Read the model definition and answer for the solid it produces. Units are mm, in the model's axes. A direction names the side the tool comes from. Give positions to 0.01 mm unless a question says otherwise; leave off trailing zeros. Loops run counter-clockwise (first coordinate to the right, second up) from the corner with the lowest first, then second, coordinate; pieces in that order, holes last.
(1) Each of these flat-tipped pins is pushed along its axis until it touches: P1, Ø2, axis at y = 0, z = 1, coming from the -X side; P2, Ø0.8, axis at x = 0, z = 1.5, coming from the +Y side; P3, Ø3, axis at y = 0, z = 1, coming from the +X side; P4, Ø6.5, axis at x = -1.5, y = 1.5, coming from the -Z side. Where does it stop, or does it pass through?
(2) Determine the mould class of faces 1 (the face through (0, 0, 2.5)), 2 (the face through (0, -1.3, 1)), 3 (the face through (-0.54, 2.44, 1.48)), 4 (the face through (0, 0, 5)) for opening direction X: pulls with the +X half, pulls with the -X half, needs draft (parallel to the pull), parting line crosses it, or undercut.
(3) Find section A-A, the plane z = 1.95. Write down the section's boundary in (x, y).
(4) Which of the six approach directions +Z, -Z, +X, -X, +Y, -Y give full straight-line access (tool end or side, diameter ignored) to faces 5 (the face through (2, 0, 0)), 6 (the face through (1.3, 0, 1))?
(5) Straight lines are drawn through the part: probe 1 along X at (y, z) = (0.25, 0.5); probe 2 along Y at (x, z) = (1, 2.05); probe 3 along X at (y, z) = (0.75, 1.4). For each, find the intervals that lie inside material, in ascending order.
```python
from build123d import *

# Parameters (mm, degrees)
F0_R     = 7.5
F1_DEPTH = 5
F2_R     = 4.99999
F3_W     = 2.6
F3_H     = 2.6
F4_DEPTH = 2.5
F5_R     = 7.5
F5_R_2   = 2.5
F6_DEPTH = 3


# Not quite as in the source:
# - a fillet or chamfer is up to 0.001 mm smaller than in the source, because OpenCascade refuses the exact size


with BuildPart() as f1:
    # F0 (on Top) → F1 (new body)
    with BuildSketch(Plane.XY):
        Circle(F0_R)
    extrude(amount=F1_DEPTH)

    # F2 (radius 5 in the source; OpenCascade refuses exactly that, so slightly less here)
    f2_edges = [f1.edges().sort_by_distance(p)[0] for p in [
        (-7.5, 0, 5),
    ]]
    fillet(f2_edges, radius=F2_R)

    # F3 (on face) → F4 (cut)
    with BuildSketch(Plane(origin=(0, 0, 0), x_dir=(1, 0, 0), z_dir=(0, 0, -1))):
        Rectangle(F3_W, F3_H)
    extrude(amount=-F4_DEPTH, mode=Mode.SUBTRACT)

    # F5 (on face) → F6 (cut)
    with BuildSketch(Plane(origin=(0, 0, 0), x_dir=(1, 0, 0), z_dir=(0, 0, -1))):
        Circle(F5_R)
        Circle(F5_R_2, mode=Mode.SUBTRACT)
    extrude(amount=-F6_DEPTH, mode=Mode.SUBTRACT)


solid = f1.part
```
Entries:
1. P1: stops at x = -2.5
1. P2: stops at y = 2.5
1. P3: stops at x = 2.5
1. P4: stops at z = 0
2. face 1: undercut
2. face 2: undercut
2. face 3: parting line crosses it
2. face 4: needs draft
3. outline: circle Ø5 at (0, 0); hole (-1.3, -1.3) - (1.3, -1.3) - (1.3, 1.3) - (-1.3, 1.3) - close
4. face 5: -Z, +X, -X, +Y, -Y
4. face 6: -Z
5. probe 1: x = -2.49 to -1.3, 1.3 to 2.49
5. probe 2: y = -2.29 to -1.3, 1.3 to 2.29
5. probe 3: x = -2.38 to -1.3, 1.3 to 2.38
